Design review of the part built by this model. Coordinates are the model's own, in mm. Face numbers are marked on the shaded views. A direction names the side the tool comes from. Round coordinates to 2 decimals unless told otherwise and drop trailing zeros. Order: outer loops, then holes, each group sorted by start corner. A loop starts at its lowest first (then second) coordinate and runs counter-clockwise, first axis right, second up.
from build123d import *

# Parameters (mm, degrees)
SKETCH1_R           = 19
BOSS_EXTRUDE1_DEPTH = 10
SKETCH2_R           = 10
CUT_EXTRUDE1_DEPTH  = 2
FILLET1_R           = 1
SKETCH3_W           = 1
SKETCH3_H           = 4
FILLET2_R           = 0.45


with BuildPart() as part:
    # Sketch1 → Boss-Extrude1 (new body)
    with BuildSketch(Plane.XY):
        Circle(SKETCH1_R)
    extrude(amount=BOSS_EXTRUDE1_DEPTH)

    # Sketch2 → Cut-Extrude1 (cut)
    with BuildSketch(Plane.XY.offset(10)):
        Circle(SKETCH2_R)
    extrude(amount=-CUT_EXTRUDE1_DEPTH, mode=Mode.SUBTRACT)

    # Fillet1
    fillet1_edges = [part.edges().sort_by_distance(p)[0] for p in [
        (-19, 0, 10),
        (-10, 0, 8),
        (-10, 0, 10),
    ]]
    fillet(fillet1_edges, radius=FILLET1_R - 0.0001)  # a hair under: the kernel refuses the full size

    # Sketch3 → Cut-Revolve1 (revolve, cut)
    with BuildSketch(Plane(origin=(0, 0, 0), x_dir=(1, 0, 0), z_dir=(0, 1, 0)), mode=Mode.PRIVATE) as cut_revolve1_sk:
        with Locations((-19, -4.5)):
            Rectangle(SKETCH3_W, SKETCH3_H)
    revolve(cut_revolve1_sk.sketch.rotate(Axis((0, 0, 0), (0, 0, 1)), 180), axis=Axis((0, 0, 0), (0, 0, 1)), mode=Mode.SUBTRACT)

    # Fillet2
    fillet2_edges = [part.edges().sort_by_distance(p)[0] for p in [
        (-18.5, 0, 6.5),
        (-18.5, 0, 2.5),
    ]]
    fillet(fillet2_edges, radius=FILLET2_R)


solid = part.part
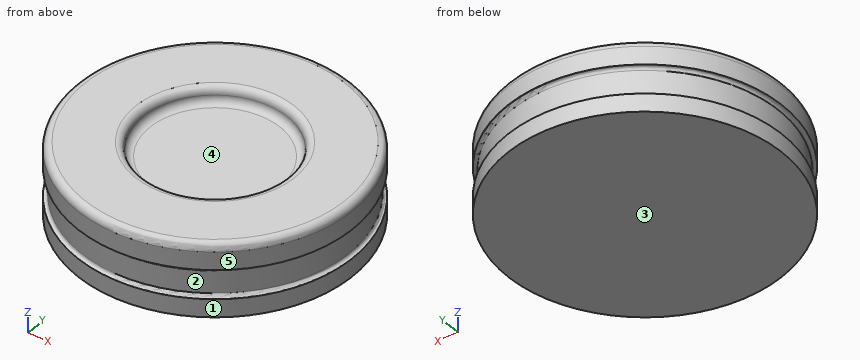
1) Take a section at D-D on z = 5. Give the boundary of the cut face in (x, y).
Results:
outline: circle Ø37 at (0, 0)
2) Take a section at C-C on z = 7.5. Give the boundary of the cut face in (x, y).
Results:
outline: circle Ø38 at (0, 0)
3) Clearance check with flat-ended pins moving along their axes: P1, Ø3, axis at x = 2.5, y = 15, coming from the -Z side; P2, Ø2, axis at x = -11.5, z = 7.5, coming from the -Y side; P3, Ø4, axis at x = -9, z = 2.5, coming from the -Y side; P4, Ø1.5, axis at y = -9, z = 8, coming from the -X side. State where each tip first meets the part, or that it passes through.
Results:
P1: stops at z = 0
P2: stops at y = -15.84
P3: stops at y = -17.66
P4: stops at x = -17.12
4) For the marked faces 4 and 5, list the 3-axis set-ups (+Z, -Z, +X, -X, +Y, -Y) from which the entire face can be reached by the end or side of a thin tool; tool diameter is ignored.
Results:
face 4: +Z
face 5: +Z, -Z
5) The part is to be moulded in two halves that separate along Z. For the marked faces 1, 2 and 3, say which applies: released by +Z, released by -Z, zero draft, split by the parting line, or undercut.
Results:
face 1: zero draft
face 2: undercut
face 3: released by -Z
6) To check wall thickness, follow line 1 along Y through (x, z) = (0, 9); line 2 along Z through (x, y) = (-2, -6); line 3 along Z through (x, y) = (16, -9.5). State the ranges of each line that lie inside material, in increasing order.
Results:
line 1: y = -19 to -10, 10 to 19
line 2: z = 0 to 8
line 3: z = 0 to 2.66, 6.34 to 9.79
